```python
from build123d import *

# Parameters (mm, degrees)
SKETCH_1_W          = 20
SKETCH_1_H          = 20
SKETCH_1_W_2        = 16
SKETCH_1_H_2        = 16
EXTRUDE_1_DEPTH     = 560
SKETCH_3_R          = 2.2
CUT_EXTRUDE_2_DEPTH = 560
SKETCH_4_R          = 2.2
CUT_EXTRUDE_3_DEPTH = 560


with BuildPart() as part:
    # ｽｹｯﾁ1 → ﾎﾞｽ - 押し出し1 (new body)
    with BuildSketch(Plane.XY):
        Rectangle(SKETCH_1_W, SKETCH_1_H)
        Rectangle(SKETCH_1_W_2, SKETCH_1_H_2, mode=Mode.SUBTRACT)
    extrude(amount=EXTRUDE_1_DEPTH)

    # ｽｹｯﾁ3 → ｶｯﾄ - 押し出し2 (cut)
    with BuildSketch(Plane(origin=(10, 0, 0), x_dir=(0, 0, -1), z_dir=(1, 0, 0))):
        with Locations((-530, 0)):
            Circle(SKETCH_3_R)
        with Locations((-30, 0)):
            Circle(SKETCH_3_R)
    extrude(amount=-CUT_EXTRUDE_2_DEPTH, mode=Mode.SUBTRACT)

    # ｽｹｯﾁ4 → ｶｯﾄ - 押し出し3 (cut)
    with BuildSketch(Plane(origin=(0, 10, 0), x_dir=(1, 0, 0), z_dir=(0, 1, 0))):
        with Locations((0, -550)):
            Circle(SKETCH_4_R)
        with Locations((0, -10)):
            Circle(SKETCH_4_R)
    extrude(amount=-CUT_EXTRUDE_3_DEPTH, mode=Mode.SUBTRACT)


solid = part.part
```
Can you work these out from the model? Positions are in its coordinate system, mm. A direction names the side the tool comes from. Give positions to 0.01 mm unless a question says otherwise; leave off trailing zeros. Loops run counter-clockwise (first coordinate to the right, second up) from the corner with the lowest first, then second, coordinate; pieces in that order, holes last. Notation, with made-up numbers: M 75.25,71.5 L 101.25,71.5 A20 cw 101.25,108.5 Z; hole C 36.5,74.5 d2. An arc over 180 degrees is marked long. One line per item, written item: value.
(1) Suppose I cut it at A-A on z = 351.5. List the corners of the cut face in (x, y) for me, plus the area to 3 significant figures.
Returned:
outline: M -10,-10 L 10,-10 L 10,10 L -10,10 Z; hole M -8,-8 L 8,-8 L 8,8 L -8,8 Z
area: 144 mm^2
(2) Which directions (+Z, -Z, +X, -X, +Y, -Y) give clear straight access to the entire face, cutting with the end or side of a thin tool? Please do faces 5 (the face through (-10, 0, 276)), 6 (the face through (-8, 0, 276)).
Returned:
face 5: +Z, -Z, -X, +Y, -Y
face 6: +Z, -Z
(3) We'd pull the mould along Y, two halves only. Please class faces 1 (the face through (0, 10, 276)), 2 (the face through (0, -10, 276)), 3 (the face through (-9, 0, 0)), 4 (the face through (0, 8, 276)): released by +Y, released by -Y, zero draft, split by the parting line, or undercut.
Returned:
face 1: released by +Y
face 2: released by -Y
face 3: zero draft
face 4: undercut
(4) Will this pin go through, and if not, where does the flat tip stop? pin 1 (2.5 mm diameter, centred on y = 0, z = 30, fed in from -X).
Returned:
pin 1: through
(5) I need wall thicknesses on line 1 (Z direction, x = 0, y = -8.8); line 2 (X direction, y = 6.5, z = 373). Which ranges of each line are inside material? Lowest first, please.
Returned:
line 1: 0 to 7.8, 12.2 to 547.8, 552.2 to 560
line 2: -10 to -8, 8 to 10
